The model under review builds one solid part; all positions refer to its coordinate system, in mm. Face numbers are marked on the shaded views. A direction names the side the tool comes from. Round coordinates to 2 decimals unless told otherwise and drop trailing zeros. Order: outer loops, then holes, each group sorted by start corner. A loop starts at its lowest first (then second) coordinate and runs counter-clockwise, first axis right, second up.
```python
from build123d import *

# Parameters (mm, degrees)
F1_DEPTH  = 80
F3_DEPTH  = 25
F4_R      = 7.5
F5_DEPTH  = 50
F6_R      = 7.5
F7_DEPTH  = 25
F9_W      = 50
F9_H      = 15
F10_DEPTH = 25
F11_R     = 7.5
F12_DEPTH = 25


with BuildPart() as f1:
    # F0 (on Front) → F1 (new body)
    with BuildSketch(Plane.XZ):
        Polygon((0, 30), (0, 0), (15, 0), (15, 15), (65, 15), (65, 0), (80, 0), (80, 30), align=None)
    extrude(amount=F1_DEPTH)

    # F2 (on face) → F3 (join)
    with BuildSketch(Plane(origin=(0, 0, 0), x_dir=(-1, 0, 0), z_dir=(0, 1, 0))):
        Polygon((-100, 0), (0, 0), (20, 0), (20, 80), (-100, 80), align=None)
    extrude(amount=F3_DEPTH)

    # F4 (on face) → F5 (join)
    with BuildSketch(Plane.XZ):
        with BuildLine():
            Line((20, 30), (40, 30))
            Line((40, 30), (60, 30))
            Line((60, 30), (60, 60))
            ThreePointArc((60, 60), (40, 80), (20, 60))
            Line((20, 60), (20, 30))
        make_face()
        with Locations((40, 60)):
            Circle(F4_R, mode=Mode.SUBTRACT)
    extrude(amount=F5_DEPTH)

    # F6 (on face) → F7 (cut, through all)
    with BuildSketch(Plane.XZ):
        with Locations((80, 60)):
            Circle(F6_R)
        with Locations((0, 60)):
            Circle(F6_R)
    extrude(amount=-F7_DEPTH, mode=Mode.SUBTRACT)

    # F9 (on face) → F10 (cut, through all)
    with BuildSketch(Plane.XZ):
        with Locations((40, 7.5)):
            Rectangle(F9_W, F9_H)
    extrude(amount=-F10_DEPTH, mode=Mode.SUBTRACT)

    # F11 (on face) → F12 (cut, through all)
    with BuildSketch(Plane.XZ):
        with Locations((40, 60)):
            Circle(F11_R)
    extrude(amount=-F12_DEPTH, mode=Mode.SUBTRACT)


solid = f1.part
```
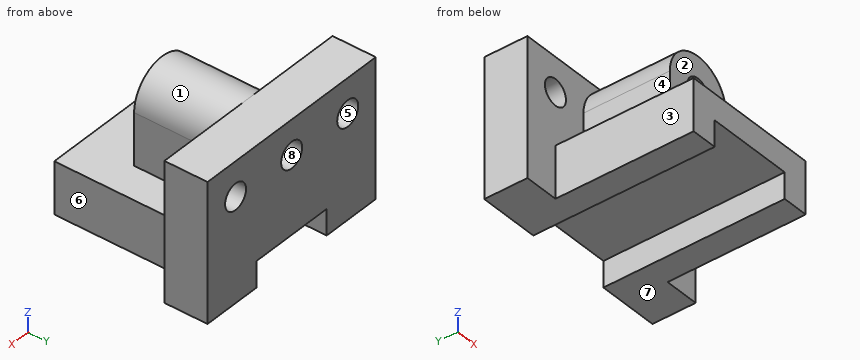
(1) Consider section C-C (y = -17). Write out the cut boundary in (x, z), and give its area (3 significant figures).
Data:
outline: (0, 0) - (15, 0) - (15, 15) - (65, 15) - (65, 0) - (80, 0) - (80, 30) - (60, 30) - (60, 60) arc R20 ccw to (20, 60) - (20, 30) - (0, 30) - close; hole circle Ø15 at (40, 60)
area: 3,300 mm2
(2) Consider section B-B (y = 13). Write out the cut boundary in (x, z).
Data:
outline: (-20, 0) - (15, 0) - (15, 15) - (65, 15) - (65, 0) - (100, 0) - (100, 80) - (-20, 80) - close; hole circle Ø15 at (0, 60); hole circle Ø15 at (40, 60); hole circle Ø15 at (80, 60)
(3) Insertion check: pin 1 (24 mm diameter, centred on y = -14.5, z = 48, fed in from -X); pin 2 (19.5 mm diameter, centred on x = 40, z = 60, fed in from +Y); pin 3 (6 mm diameter, centred on x = 18.5, y = -56, fed in from -Z); pin 4 (15 mm diameter, centred on y = -20.5, z = 16.5, fed in from -X). Each pin has a flat end and moves straight along its axis. Give the tip position at first contact, or say it passes through.
Data:
pin 1: stops at x = 20
pin 2: stops at y = 25
pin 3: stops at z = 15
pin 4: stops at x = 0
(4) Consider section A-A (z = 11). Write out the cut boundary in (x, y), and give its area (3 significant figures).
Data:
outline: (-20, 0) - (0, 0) - (0, -80) - (15, -80) - (15, 25) - (-20, 25) - close; (65, -80) - (80, -80) - (80, 0) - (100, 0) - (100, 25) - (65, 25) - close
area: 4,150 mm2
(5) Consider section D-D (z = 40.5). Write out the cut boundary in (x, y).
Data:
outline: (-20, 0) - (20, 0) - (20, -50) - (60, -50) - (60, 0) - (100, 0) - (100, 25) - (-20, 25) - close
(6) Draft analysis for pull direction Z (two halves, no side actions). For the marked faces 5, 6, 7 and 8, state which applies: pulls with the +Z half, pulls with the -Z half, needs draft (parallel to the pull), parting line crosses it, or undercut.
Data:
face 5: undercut
face 6: needs draft
face 7: pulls with the -Z half
face 8: undercut
(7) For the marked faces 1, 2, 3 and 4, list the 3-axis set-ups (+Z, -Z, +X, -X, +Y, -Y) from which the entire face can be reached by the end or side of a thin tool; tool diameter is ignored.
Data:
face 1: +Z, -Y
face 2: +Z, +X, -X, -Y
face 3: +Z, -Z, -X, -Y
face 4: +Z, -X, -Y
(8) To check wall thickness, follow probe 1 along X at (y, z) = (7, 55); probe 2 along Z at (x, y) = (40, -17); probe 3 along X at (y, z) = (3, 54). State the ranges of each line that lie inside material, in increasing order.
Data:
probe 1: x = -20 to -5.59, 5.59 to 34.41, 45.59 to 74.41, 85.59 to 100
probe 2: z = 15 to 52.5, 67.5 to 80
probe 3: x = -20 to -4.5, 4.5 to 35.5, 44.5 to 75.5, 84.5 to 100
